```python
from build123d import *

# Parameters (mm, degrees)
BOSS_EXTRUDE1_DEPTH = 50.8
SKETCH2_R           = 2.921
BOSS_EXTRUDE2_DEPTH = 4.445
FILLET1_R           = 0.254
SKETCH3_R           = 1.651
CUT_EXTRUDE1_DEPTH  = 55.746198624
SKETCH4_R           = 2.921
BOSS_EXTRUDE3_DEPTH = 4.445
FILLET2_R           = 0.254
SKETCH5_R           = 1.651
CUT_EXTRUDE2_DEPTH  = 55.746198624


with BuildPart() as part:
    # Sketch1 → Boss-Extrude1 (new body)
    with BuildSketch(Plane(origin=(0, 0, 0), x_dir=(1, 0, 0), z_dir=(0, 1, 0))):
        Polygon((0, 0), (11.43, 0), (11.43, -2.286), (16.9926, -2.286), (16.9926, -6.858), (6.223, -6.858), (6.223, -3.302), (-6.223, -3.302), (-6.223, -6.858), (-16.9926, -6.858), (-16.9926, -2.286), (-11.43, -2.286), (-11.43, 0), align=None)
    extrude(amount=BOSS_EXTRUDE1_DEPTH)

    # Sketch2 → Boss-Extrude2 (add)
    with BuildSketch(Plane(origin=(0, 0, 0), x_dir=(-1, 0, 0), z_dir=(0, 0, -1))):
        with Locations(Location((0, 15.24, 0), (0, 0, 180))):
            Circle(SKETCH2_R)
    extrude(amount=BOSS_EXTRUDE2_DEPTH)

    # Fillet1
    fillet1_edges = [part.edges().sort_by_distance(p)[0] for p in [
        (-2.921, 15.24, -4.445),
    ]]
    fillet(fillet1_edges, radius=FILLET1_R)

    # Sketch3 → Cut-Extrude1 (cut, through all)
    with BuildSketch(Plane(origin=(0, 0, -4.445), x_dir=(-1, 0, 0), z_dir=(0, 0, -1))):
        with Locations((0, 15.24)):
            Circle(SKETCH3_R)
    extrude(amount=-CUT_EXTRUDE1_DEPTH, mode=Mode.SUBTRACT)

    # Sketch4 → Boss-Extrude3 (add)
    with BuildSketch(Plane(origin=(0, 0, 0), x_dir=(-1, 0, 0), z_dir=(0, 0, -1))):
        with Locations(Location((0, 35.56, 0), (0, 0, 180))):
            Circle(SKETCH4_R)
    extrude(amount=BOSS_EXTRUDE3_DEPTH)

    # Fillet2
    fillet2_edges = [part.edges().sort_by_distance(p)[0] for p in [
        (-2.921, 35.56, -4.445),
    ]]
    fillet(fillet2_edges, radius=FILLET2_R)

    # Sketch5 → Cut-Extrude2 (cut, through all)
    with BuildSketch(Plane(origin=(0, 0, -4.445), x_dir=(-1, 0, 0), z_dir=(0, 0, -1))):
        with Locations((0, 35.56)):
            Circle(SKETCH5_R)
    extrude(amount=-CUT_EXTRUDE2_DEPTH, mode=Mode.SUBTRACT)


solid = part.part
```
Can you work these out from the model? Positions are in its coordinate system, mm. A direction names the side the tool comes from. Round coordinates to 2 decimals unless told otherwise and drop trailing zeros. Loops run counter-clockwise (first coordinate to the right, second up) from the corner with the lowest first, then second, coordinate; pieces in that order, holes last. Notation, with made-up numbers: M 44.25,7 L 61.25,7 A21 ccw 61.25,15 Z; hole C 68,-26 d7. An arc over 180 degrees is marked long. Write item = value, one per line. Start each with the question number.
(1) Suppose I cut it at B-B on y = 35.56. Write out the boundary of the cut face in (x, z) (3 decimals), plus the area to 3 significant figures.
(2) I need wall thicknesses on line 1 along X through (y, z) = (8.5, 5.5); line 2 along Y through (x, z) = (0, -1); line 3 along Y through (x, z) = (0, 0.25). Which ranges of each line are inside material? Lowest first, please.
(3) Suppose I cut it at C-C on y = 21.5. Write out the boundary of the cut face in (x, z), plus the area to 3 significant figures.
(4) Suppose I cut it at D-D on z = -0.5. Write out the boundary of the cut face in (x, y), plus the area to 3 significant figures.
(5) Which directions (+Z, -Z, +X, -X, +Y, -Y) give clear straight access to the entire face, cutting with the end or side of a thin tool? Please do faces 1 (the face through (-0.38, 32.664, -2.066)), 2 (the face through (11.43, 25, 1)), 3 (the face through (-14, 25, 2.286)), 4 (the face through (0, 25, 3.302)), 5 (the face through (1, 34, -4.445)).
(6) Suppose I cut it at A-A on z = 5.5. Write out the boundary of the cut face in (x, y).
(7) I'm going to push flat-ended pins straight in: P1, Ø3, axis at x = -14.5, y = 15, coming from the -Z side; P2, Ø4, axis at x = 3.5, y = 6.5, coming from the +Z side; P3, Ø6, axis at x = 13.5, y = 21, coming from the -Z side; P4, Ø2, axis at x = 0, y = 35.56, coming from the -Z side. Where does each tip first touch, or does it pass through?
(8) If we mould it in two halves opening along Y, with no side actions, what happens to faces 6 (the face through (0, 50.8, 3)), 7 (the face through (-0.6, 18.1, -2.1)), 8 (the face through (6.223, 25, 5))? For each: released by +Y, released by -Y, zero draft, split by the parting line, or undercut.
Answer block:
q1.outline = M -16.993,2.286 L -11.43,2.286 L -11.43,0 L -2.921,0 L -2.921,-4.191 A0.254 ccw -2.667,-4.445 L -1.651,-4.445 L -1.651,3.302 L -6.223,3.302 L -6.223,6.858 L -16.993,6.858 Z; M 1.651,-4.445 L 2.667,-4.445 A0.254 ccw 2.921,-4.191 L 2.921,0 L 11.43,0 L 11.43,2.286 L 16.993,2.286 L 16.993,6.858 L 6.223,6.858 L 6.223,3.302 L 1.651,3.302 Z
q1.area = 164 mm²
q2.line_1 = -16.99 to -6.22, 6.22 to 16.99
q2.line_2 = 12.32 to 13.59, 16.89 to 18.16, 32.64 to 33.91, 37.21 to 38.48
q2.line_3 = 0 to 13.59, 16.89 to 33.91, 37.21 to 50.8
q3.outline = M -16.99,2.29 L -11.43,2.29 L -11.43,0 L 11.43,0 L 11.43,2.29 L 16.99,2.29 L 16.99,6.86 L 6.22,6.86 L 6.22,3.3 L -6.22,3.3 L -6.22,6.86 L -16.99,6.86 Z
q3.area = 163 mm²
q4.outline = C 0,15.24 d5.84; C 0,35.56 d5.84; hole C 0,15.24 d3.3; hole C 0,35.56 d3.3
q4.area = 36.5 mm²
q5.face_1 = -Z
q5.face_2 = -Z, +X, +Y, -Y
q5.face_3 = -Z, -X, +Y, -Y
q5.face_4 = +Z, +Y, -Y
q5.face_5 = -Z, +X, -X, +Y, -Y
q6.outline = M -16.99,0 L -6.22,0 L -6.22,50.8 L -16.99,50.8 Z; M 6.22,0 L 16.99,0 L 16.99,50.8 L 6.22,50.8 Z
q7.P1 = 2.29
q7.P2 = 3.3
q7.P3 = 0
q7.P4 = through
q8.face_6 = released by +Y
q8.face_7 = undercut
q8.face_8 = zero draft
